Could you check a few things on this model? Use its own coordinates, in mm. Give positions to 0.01 mm unless a question says otherwise; leave off trailing zeros. Order: outer loops, then holes, each group sorted by start corner. A loop starts at its lowest first (then second) coordinate and runs counter-clockwise, first axis right, second up. Notation, with made-up numbers: (-11.75, 44) -> (3.25, 44) arc R15 cw to (3.25, 55) -> close; hole circle Ø7 at (50, 33.5). An arc over 180 degrees is marked (long way). One line per item, written item: value.
```python
from build123d import *

# Parameters (mm, degrees)
SKETCH1_W                  = 130
SKETCH1_H                  = 150
BOSS_EXTRUDE1_DEPTH        = 3
F_10_0_10_DIAMETER_HOLE2_D = 10
F_14_0_14_DIAMETER_HOLE1_D = 14
F_5_0_5_DIAMETER_HOLE1_D   = 5
F_10_0_10_DIAMETER_HOLE1_D = 10
F_9_0_9_DIAMETER_HOLE1_D   = 9
F_5_0_5_DIAMETER_HOLE2_D   = 5
SKETCH15_W                 = 130
SKETCH15_H                 = 30
CUT_EXTRUDE1_DEPTH         = 199.517001791
SKETCH16_R                 = 2.35
CUT_EXTRUDE2_DEPTH         = 199.517001791


with BuildPart() as part:
    # Sketch1 → Boss-Extrude1 (new body)
    with BuildSketch(Plane(origin=(0, 0, 0), x_dir=(1, 0, 0), z_dir=(0, 1, 0))):
        with Locations((65, -75)):
            Rectangle(SKETCH1_W, SKETCH1_H)
    extrude(amount=BOSS_EXTRUDE1_DEPTH)

    # Ø10.0 (10) Diameter Hole2 (through all)
    with Locations(Plane(origin=(0, 3, 0), x_dir=(1, 0, 0), z_dir=(0, 1, 0))):
        with Locations((40, -128), (98, -128), (74, -66)):
            Hole(F_10_0_10_DIAMETER_HOLE2_D / 2)

    # Ø14.0 (14) Diameter Hole1 (through all)
    with Locations(Plane(origin=(0, 3, 0), x_dir=(1, 0, 0), z_dir=(0, 1, 0))):
        with Locations((16, -16), (114, -16)):
            Hole(F_14_0_14_DIAMETER_HOLE1_D / 2)

    # Ø5.0 (5) Diameter Hole1 (through all)
    with Locations(Plane(origin=(0, 3, 0), x_dir=(1, 0, 0), z_dir=(0, 1, 0))):
        with Locations((4.686291501, -27.313708499), (4.686291501, -4.686291501), (27.313708499, -4.686291501), (27.313708499, -27.313708499), (102.686291501, -27.313708499), (125.313708499, -27.313708499), (125.313708499, -4.686291501), (102.686291501, -4.686291501)):
            Hole(F_5_0_5_DIAMETER_HOLE1_D / 2)

    # Ø10.0 (10) Diameter Hole1 (through all)
    with Locations(Plane(origin=(0, 3, 0), x_dir=(1, 0, 0), z_dir=(0, 1, 0))):
        with Locations((86, -135), (86, -80)):
            Hole(F_10_0_10_DIAMETER_HOLE1_D / 2)

    # Ø9.0 (9) Diameter Hole1 (through all)
    with Locations(Plane(origin=(0, 3, 0), x_dir=(1, 0, 0), z_dir=(0, 1, 0))):
        with Locations((65, -16)):
            Hole(F_9_0_9_DIAMETER_HOLE1_D / 2)

    # Ø5.0 (5) Diameter Hole2 (through all)
    with Locations(Plane(origin=(0, 3, 0), x_dir=(1, 0, 0), z_dir=(0, 1, 0))):
        with Locations((53.686291501, -27.313708499), (76.313708499, -27.313708499), (76.313708499, -4.686291501), (53.686291501, -4.686291501)):
            Hole(F_5_0_5_DIAMETER_HOLE2_D / 2)

    # Sketch15 → Cut-Extrude1 (cut, through all)
    with BuildSketch(Plane(origin=(0, 0, 0), x_dir=(1, 0, 0), z_dir=(0, 1, 0))):
        with Locations((65, -15)):
            Rectangle(SKETCH15_W, SKETCH15_H)
    extrude(amount=CUT_EXTRUDE1_DEPTH, mode=Mode.SUBTRACT)

    # Sketch16 → Cut-Extrude2 (cut, through all)
    with BuildSketch(Plane(origin=(0, 0, 0), x_dir=(1, 0, 0), z_dir=(0, 1, 0))):
        with Locations(Location((89.95, -37.25, 0), (0, 0, 90))):
            Circle(SKETCH16_R)
        with Locations(Location((118.05, -37.25, 0), (0, 0, 90))):
            Circle(SKETCH16_R)
        with Locations(Location((104, -40.25, 0), (0, 0, 90))):
            Circle(SKETCH16_R)
        with Locations(Location((11.95, -37.25, 0), (0, 0, 90))):
            Circle(SKETCH16_R)
        with Locations(Location((40.05, -37.25, 0), (0, 0, 90))):
            Circle(SKETCH16_R)
        with Locations(Location((26, -40.25, 0), (0, 0, 90))):
            Circle(SKETCH16_R)
    extrude(amount=CUT_EXTRUDE2_DEPTH, mode=Mode.SUBTRACT)


solid = part.part
```
1) Suppose I cut it at C-C, the plane y = 1.55. State how many separate pieces and enclosed holes the cut face has, then the cut area to 3 significant figures.
Answer below:
separate pieces: 1
enclosed holes: 11
area: 15,100 mm2
2) Suppose I cut it at D-D, the plane x = 85. Write out the boundary of the cut face in (y, z), then the cut area to 3 significant figures.
Answer below:
outline: (0, 30) -> (3, 30) -> (3, 75.1) -> (0, 75.1) -> close; (0, 84.9) -> (3, 84.9) -> (3, 130.1) -> (0, 130.1) -> close; (0, 139.9) -> (3, 139.9) -> (3, 150) -> (0, 150) -> close
area: 301 mm2
3) We'd pull the mould along X, two halves only. Please class faces 1 (the flat face through (64, 1, 30)), 2 (the cylindrical face through (102.018, 1.479, 38.987)), 3 (the cylindrical face through (45, 1, 128)), 4 (the flat face through (130, 1, 91)): +X half, -X half, draft (parallel to the pull), parting line (faces both ways), or undercut.
Answer below:
face 1: draft
face 2: undercut
face 3: undercut
face 4: +X half
4) Suppose I cut it at A-A, the plane z = 66. Write out the boundary of the cut face in (x, y), then the cut area to 3 significant figures.
Answer below:
outline: (0, 0) -> (69, 0) -> (69, 3) -> (0, 3) -> close; (79, 0) -> (130, 0) -> (130, 3) -> (79, 3) -> close
area: 360 mm2
5) If I drill on line 1 along X through (y, z) = (2, 37.25); line 2 along X through (y, z) = (2.05, 40.25); line 3 along Z through (x, y) = (102.5, 1.35), over which ranges is the centre line in solid material (lowest first)?
Answer below:
line 1: x = 0 to 9.6, 14.3 to 37.7, 42.4 to 87.6, 92.3 to 115.7, 120.4 to 130
line 2: x = 0 to 23.65, 28.35 to 101.65, 106.35 to 130
line 3: z = 30 to 38.44, 42.06 to 125.82, 130.18 to 150
6) Suppose I cut it at B-B, the plane x = 11.95. Write out the boundary of the cut face in (y, z).
Answer below:
outline: (0, 30) -> (3, 30) -> (3, 34.9) -> (0, 34.9) -> close; (0, 39.6) -> (3, 39.6) -> (3, 150) -> (0, 150) -> close
